Print and shaded views of the part. All mm, measured from the part's lowest x, y and z. A direction names the side the tool comes from. Coordinates: 2 decimals unless noted, no trailing zeros. Order: outer loops, then holes, each group sorted by start corner. A loop starts at its lowest first (then second) coordinate and runs counter-clockwise, first axis right, second up. Notation, with made-up numbers: (45.5, 89) -> (100.5, 89) arc R13 cw to (100.5, 101) -> close; hole circle Ø6 at (35.25, 10). An arc over 180 degrees is marked (long way). Return JSON: item names as keys, results as strings. Group by question number.
1) Flat gauge pin, fed straight in: pin 1 (1.2 mm diameter, centred on x = 2, y = 2, fed in from +Z). Where does the tip first touch, or does it go through?
2) Which spindle directions (+Z, -Z, +X, -X, +Y, -Y) get a long thin tool onto all of the face, cutting with end or side? Do the marked faces 1 and 2. Say none if no direction does.
3) Probe line 1 (Y direction, x = 2, z = 1.55); line 2 (X direction, y = 1.25, z = 0.2); line 3 (Y direction, x = 8.25, z = 1.45). List the from-to ranges inside material, lowest first.
4) Cut at D-D (x = 5). Write the cut outline in (y, z), and give its area (3 significant figures).
5) Cut at B-B (y = 2). Write the cut outline in (x, z).
6) Pull direction X, two halves, no side cores. Call the marked faces 3, 4 and 5: +X half, -X half, draft (parallel to the pull), parting line (faces both ways), or undercut.
7) Cut at A-A (x = 17.5). Write the cut outline in (y, z), and give its area (3 significant figures).
8) Cut at C-C (z = 0.95). Write the cut outline in (x, y), and give its area (3 significant figures).
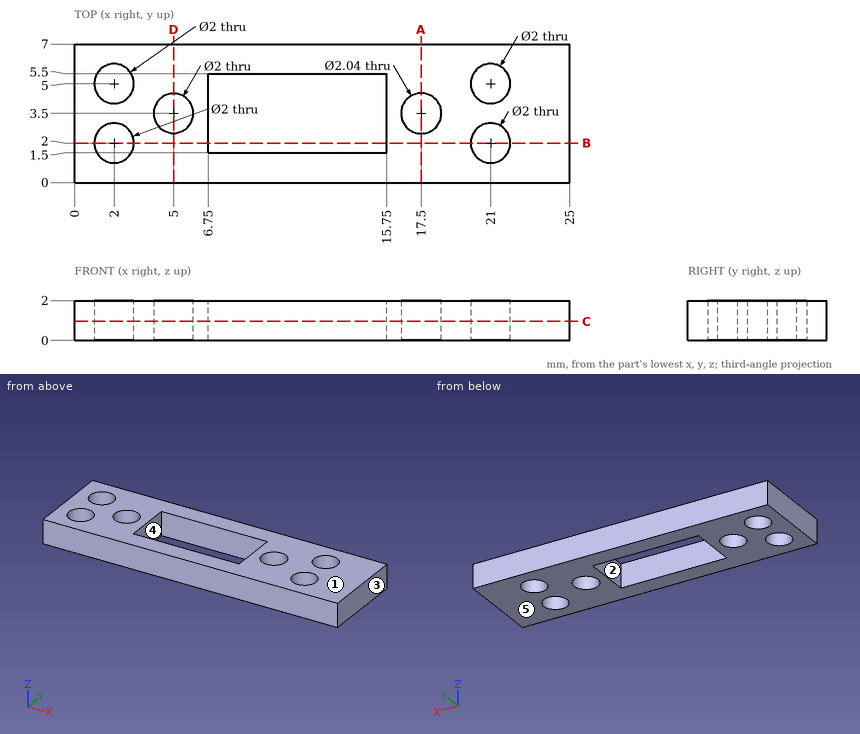
Answers below:
{
 "1": {"pin 1": "passes through"},
 "2": {"face 1": "+Z, +X, -X, +Y, -Y", "face 2": "+Z, -Z"},
 "3": {"line 1": "y = 0 to 1, 3 to 4, 6 to 7", "line 2": "x = 0 to 1.34, 2.66 to 20.34, 21.66 to 25", "line 3": "y = 0 to 1.5, 5.5 to 7"},
 "4": {"outline": "(0, 0) -> (2.5, 0) -> (2.5, 2) -> (0, 2) -> close; (4.5, 0) -> (7, 0) -> (7, 2) -> (4.5, 2) -> close", "area": "10.0 mm^2"},
 "5": {"outline": "(0, 0) -> (1, 0) -> (1, 2) -> (0, 2) -> close; (3, 0) -> (6.75, 0) -> (6.75, 2) -> (3, 2) -> close; (15.75, 0) -> (20, 0) -> (20, 2) -> (15.75, 2) -> close; (22, 0) -> (25, 0) -> (25, 2) -> (22, 2) -> close"},
 "6": {"face 3": "+X half", "face 4": "undercut", "face 5": "draft"},
 "7": {"outline": "(0, 0) -> (2.48, 0) -> (2.48, 2) -> (0, 2) -> close; (4.52, 0) -> (7, 0) -> (7, 2) -> (4.52, 2) -> close", "area": "9.92 mm^2"},
 "8": {"outline": "(0, 0) -> (25, 0) -> (25, 7) -> (0, 7) -> close; hole circle Ø2 at (2, 2); hole circle Ø2 at (2, 5); hole circle Ø2 at (5, 3.5); hole (6.75, 1.5) -> (15.75, 1.5) -> (15.75, 5.5) -> (6.75, 5.5) -> close; hole circle Ø2.04 at (17.5, 3.5); hole circle Ø2 at (21, 2); hole circle Ø2 at (21, 5)", "area": "120 mm^2"}
}
